```python
from build123d import *

# Parameters (mm, degrees)
SKETCH1_W                    = 9.525
SKETCH1_H                    = 32
BOSS_EXTRUDE1_DEPTH          = 3
SKETCH2_W                    = 11.725
SKETCH2_H                    = 34.2
SKETCH2_W_2                  = 9.525
SKETCH2_H_2                  = 32
BOSS_EXTRUDE2_DEPTH          = 11
SKETCH3_R                    = 2.3
CUT_EXTRUDE1_DEPTH           = 69.046312354
CUT_EXTRUDE1_DRAFT           = 3
CUT_EXTRUDE1_PROFILE_2_DEPTH = 69.046312354
CUT_EXTRUDE1_PROFILE_2_DRAFT = 3
MOVE_FACE1_BY                = 0.35
MOVE_FACE1_2_BY              = 0.35
MOVE_FACE1_3_BY              = 0.35
MOVE_FACE1_4_BY              = 0.35
MOVE_FACE1_5_BY              = 0.35


with BuildPart() as part:
    # Sketch1 → Boss-Extrude1 (new body)
    with BuildSketch(Plane.XY):
        with Locations((59.5125, 0)):
            Rectangle(SKETCH1_W, SKETCH1_H)
    extrude(amount=BOSS_EXTRUDE1_DEPTH)

    # Sketch2 → Boss-Extrude2 (add)
    with BuildSketch(Plane.XY.offset(3)):
        with Locations((59.5125, 0)):
            Rectangle(SKETCH2_W, SKETCH2_H)
        with Locations((59.5125, 0)):
            Rectangle(SKETCH2_W_2, SKETCH2_H_2, mode=Mode.SUBTRACT)
    extrude(amount=-BOSS_EXTRUDE2_DEPTH)


with BuildPart() as cut_extrude1_tool:
    # Sketch3 → Cut-Extrude1 (with draft: the straight prism first)
    with BuildSketch(Plane(origin=(0, 0, 0), x_dir=(-1, 0, 0), z_dir=(0, 0, -1))):
        with Locations((-59.5125, 7)):
            Circle(SKETCH3_R)
    extrude(amount=-CUT_EXTRUDE1_DEPTH)
    # Cut-Extrude1: the draft: its side faces are tilted about the plane it starts from
    cut_extrude1_sides = [cut_extrude1_tool.faces().sort_by_distance(p)[0] for p in [
        (61.8125, 7, 34.523156177),
    ]]
    draft(cut_extrude1_sides, Plane(origin=(0, 0, 0), x_dir=(-1, 0, 0), z_dir=(0, 0, -1)), CUT_EXTRUDE1_DRAFT)


with BuildPart() as part_1:
    add(part.part)

    # Cut-Extrude1: cut by cut_extrude1_tool
    add(cut_extrude1_tool.part, mode=Mode.SUBTRACT)


with BuildPart() as cut_extrude1_profile_2_tool:
    # Sketch3 → Cut-Extrude1 profile 2 (with draft: the straight prism first)
    with BuildSketch(Plane(origin=(0, 0, 0), x_dir=(-1, 0, 0), z_dir=(0, 0, -1))):
        with Locations((-59.5125, -7)):
            Circle(SKETCH3_R)
    extrude(amount=-CUT_EXTRUDE1_PROFILE_2_DEPTH)
    # Cut-Extrude1 profile 2: the draft: its side faces are tilted about the plane it starts from
    cut_extrude1_profile_2_sides = [cut_extrude1_profile_2_tool.faces().sort_by_distance(p)[0] for p in [
        (61.8125, -7, 34.523156177),
    ]]
    draft(cut_extrude1_profile_2_sides, Plane(origin=(0, 0, 0), x_dir=(-1, 0, 0), z_dir=(0, 0, -1)), CUT_EXTRUDE1_PROFILE_2_DRAFT)


with BuildPart() as part_2:
    add(part_1.part)

    # Cut-Extrude1 profile 2: cut by cut_extrude1_profile_2_tool
    add(cut_extrude1_profile_2_tool.part, mode=Mode.SUBTRACT)

    # Move Face1: a face moved inward by 0.35
    extrude(part_2.faces().sort_by_distance((59.5125, -16, -4))[0], amount=MOVE_FACE1_BY, dir=(0, -1, 0), mode=Mode.SUBTRACT)

    # Move Face1 2: a face moved inward by 0.35
    extrude(part_2.faces().sort_by_distance((54.75, 0, -4))[0], amount=MOVE_FACE1_2_BY, dir=(-1, 0, 0), mode=Mode.SUBTRACT)

    # Move Face1 3: a face moved inward by 0.35
    extrude(part_2.faces().sort_by_distance((64.275, 0, -4))[0], amount=MOVE_FACE1_3_BY, dir=(1, 0, 0), mode=Mode.SUBTRACT)

    # Move Face1 4: a face moved inward by 0.35
    extrude(part_2.faces().sort_by_distance((59.5125, 16, -4))[0], amount=MOVE_FACE1_4_BY, dir=(0, 1, 0), mode=Mode.SUBTRACT)

    # Move Face1 5: a face moved inward by 0.35
    extrude(part_2.faces().sort_by_distance((59.5125, 0, 0))[0], amount=MOVE_FACE1_5_BY, dir=(0, 0, 1), mode=Mode.SUBTRACT)


solid = part_2.part
```
Work out the finished part from the listing and answer in its coordinate system (mm). A direction names the side the tool comes from. Round coordinates to 2 decimals unless told otherwise and drop trailing zeros. Loops run counter-clockwise (first coordinate to the right, second up) from the corner with the lowest first, then second, coordinate; pieces in that order, holes last. Notation, with made-up numbers: M 8.5,56 L 61.5,56 A36 ccw 61.5,90 Z; hole C -31,74.5 d11. An arc over 180 degrees is marked long. One line per question, with ' | ' between items.
Q1. Find section C-C, the plane y = -10.5. Give the vertices of the cut face in (x, z) (3 decimals).
Conclusion:
outline: M 53.65,-8 L 54.4,-8 L 54.4,0.35 L 64.625,0.35 L 64.625,-8 L 65.375,-8 L 65.375,3 L 53.65,3 Z
Q2. Consider line 1 along Y through (x, z) = (63.5, -4.25); line 2 along X through (y, z) = (8, -1.75) (3 decimals); line 3 along Z through (x, y) = (62.25, 9). Determine where each line is inside the solid, lowest interval first. Write a range as from..to.
Conclusion:
line 1: y = -17.1..-16.35, 16.35..17.1 | line 2: x = 53.65..54.4, 64.625..65.375 | line 3: z = 0.35..3
Q3. The mould has two halves that part along Y. Classify faces 1 (the flat face through (59, 0, 3)), 2 (the flat face through (59, 17.1, -2)), 3 (the flat face through (59, 16.35, -4)): +Y half, -Y half, draft (parallel to the pull), parting line (faces both ways), or undercut.
Conclusion:
face 1: draft | face 2: +Y half | face 3: undercut
Q4. A tool of negligible diameter and unlimited length cuts with its end or side. For faces 4 (the flat face through (53.65, 0, -2)), 5 (the flat face through (54.4, 0, -4)), from which of +Z, -Z, +X, -X, +Y, -Y can it reach the whole face along a straight path? Write none if from no direction.
Conclusion:
face 4: +Z, -Z, -X, +Y, -Y | face 5: -Z
Q5. This flat-tipped pin is pushed along its axis until it touches: pin 1 Ø5 at (x, y) = (61, 6) entering from -Z. Where does it stop, or does it pass through?
Conclusion:
pin 1: stops at z = 0.35
Q6. Find section A-A, the plane z = -1. Give the vertices of the cut face in (x, y) (3 decimals), then the cut area to 3 significant figures.
Conclusion:
outline: M 53.65,-17.1 L 65.375,-17.1 L 65.375,17.1 L 53.65,17.1 Z; hole M 54.4,-16.35 L 64.625,-16.35 L 64.625,16.35 L 54.4,16.35 Z | area: 66.6 mm2
Q7. Find section B-B, the plane x = 55.75. Give the vertices of the cut face in (y, z).
Conclusion:
outline: M -17.1,-8 L -16.35,-8 L -16.35,0.35 L 16.35,0.35 L 16.35,-8 L 17.1,-8 L 17.1,3 L -17.1,3 Z
Q8. Find section D-D, the plane y = 7. Give the vertices of the cut face in (x, z) (3 decimals), then the cut area to 3 significant figures.
Conclusion:
outline: M 53.65,-8 L 54.4,-8 L 54.4,0.35 L 57.194,0.35 L 57.055,3 L 53.65,3 Z; M 61.831,0.35 L 64.625,0.35 L 64.625,-8 L 65.375,-8 L 65.375,3 L 61.97,3 Z | area: 30.9 mm2
